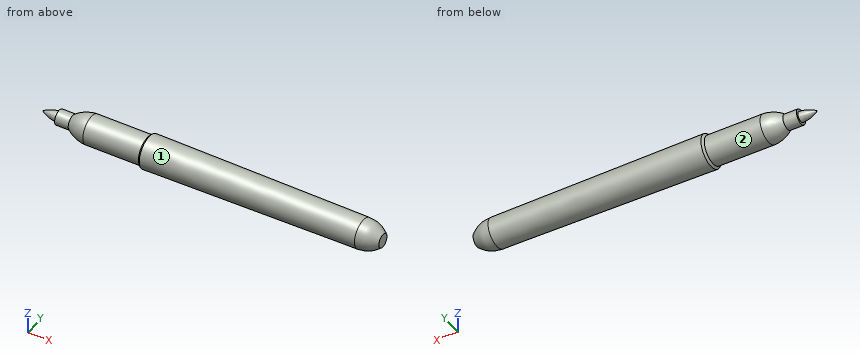
```python
from build123d import *

# Parameters (mm, degrees)
SKETCH9_W = 20.828
SKETCH9_H = 5.334
FILLET1_R = 0.127


with BuildPart() as part:
    # Sketch9 → Revolve2 (revolve)
    with BuildSketch(Plane.XY):
        with BuildLine():
            Line((-127, 0), (-121.031, 0))
            Line((-121.031, 0), (-121.031, 1.905))
            ThreePointArc((-121.031, 1.905), (-124.125234531, 1.384394498), (-127, 0.127))
            Line((-127, 0.127), (-127, 0))
        make_face()
        Polygon((-121.031, 0), (-115.951, 0), (-115.951, 2.794), (-121.031, 2.794), (-121.031, 1.905), align=None)
        with BuildLine():
            Line((-115.951, 0), (-108.966, 0))
            Line((-108.966, 0), (-108.966, 5.334))
            ThreePointArc((-108.966, 5.334), (-112.655640632, 4.606136738), (-115.951, 2.794))
            Line((-115.951, 2.794), (-115.951, 0))
        make_face()
        with Locations((-98.552, 2.667)):
            Rectangle(SKETCH9_W, SKETCH9_H)
        with BuildLine():
            Line((-88.138, 0), (-87.376, 0))
            Line((-87.376, 0), (-87.376, 6.1595))
            ThreePointArc((-87.376, 6.1595), (-87.803422559, 5.789601593), (-88.138, 5.334))
            Line((-88.138, 5.334), (-88.138, 0))
        make_face()
        Polygon((-87.376, 0), (-7.366, 0), (-7.366, 5.461), (-87.376, 6.1595), align=None)
        with BuildLine():
            Line((-7.366, 0), (0, 0))
            Line((0, 0), (0, 2.54))
            ThreePointArc((0, 2.54), (-3.396669863, 4.722549911), (-7.366, 5.461))
            Line((-7.366, 5.461), (-7.366, 0))
        make_face()
    revolve(axis=Axis((0, 0, 0), (-1, 0, 0)))

    # Fillet1
    fillet1_edges = [part.edges().sort_by_distance(p)[0] for p in [
        (-127, -0.127, 0),
    ]]
    fillet(fillet1_edges, radius=FILLET1_R)


solid = part.part
```
CAD build for the part. Positions are in the model's coordinates, mm. Face numbers are marked on the shaded views. A direction names the side the tool comes from. Coordinates: 2 decimals unless noted, no trailing zeros. Order: outer loops, then holes, each group sorted by start corner. A loop starts at its lowest first (then second) coordinate and runs counter-clockwise, first axis right, second up.
(1) Drill centre lines: L1, parallel to Z at x = -118.5, y = -0.25; L2, parallel to X at y = -0.5, z = 2; L3, parallel to Z at x = -36, y = -1.75. Where is each one in solid material? Low to high.
Solution:
L1: z = -2.78 to 2.78
L2: x = -121.03 to 0
L3: z = -5.44 to 5.44
(2) Saw through at B-B, the plane x = -19. Write the cut outline in (y, z).
Solution:
outline: circle Ø11.13 at (0, 0)
(3) Which spindle directions (+Z, -Z, +X, -X, +Y, -Y) get a long thin tool onto all of the face, cutting with end or side? Do the marked faces 1 and 2. Say none if no direction does.
Solution:
face 1: +X
face 2: -X
(4) Pin check, flat tips, straight feed: pin 1 Ø2 at (x, y) = (-51.5, 1) entering from -Z; pin 2 Ø4 at (x, z) = (-37, 2) entering from -Y; pin 3 Ø1 at (x, y) = (-32.5, -2) entering from +Z. Stop position of each tip, or through.
Solution:
pin 1: stops at z = -5.85
pin 2: stops at y = -5.72
pin 3: stops at z = 5.48
(5) Saw through at A-A, the plane x = -117. Write the cut outline in (y, z), and give its area (3 significant figures).
Solution:
outline: circle Ø5.59 at (0, 0)
area: 24.5 mm2
